Build history of the part. All positions in model axes, mm. A direction names the side the tool comes from. Round coordinates to 2 decimals unless told otherwise and drop trailing zeros. Loops run counter-clockwise (first coordinate to the right, second up) from the corner with the lowest first, then second, coordinate; pieces in that order, holes last. Notation, with made-up numbers: (53.25, 81) - (80.25, 81) arc R29 cw to (80.25, 118) - close; hole circle Ø6 at (67.5, 69). An arc over 180 degrees is marked (long way). Use a Markdown table: item, result.
from build123d import *

# Parameters (mm, degrees)
SKETCH2_W           = 60
SKETCH2_H           = 60
BOSS_EXTRUDE1_DEPTH = 15
CUT_EXTRUDE1_DEPTH  = 3
SKETCH1_R           = 2.25
BOSS_EXTRUDE2_DEPTH = 2
SKETCH4_R           = 1.25
BOSS_EXTRUDE3_DEPTH = 5
SKETCH5_R           = 2.5
BOSS_EXTRUDE4_DEPTH = 25


with BuildPart() as part:
    # Sketch2 → Boss-Extrude1 (new body)
    with BuildSketch(Plane(origin=(0, 0, 0), x_dir=(1, 0, 0), z_dir=(0, 1, 0))):
        Rectangle(SKETCH2_W, SKETCH2_H)
    extrude(amount=-BOSS_EXTRUDE1_DEPTH)

    # Sketch3 → Cut-Extrude1 (cut)
    with BuildSketch(Plane.ZY.offset(30)):
        with BuildLine():
            Line((-6.5, -7.5), (-13, -7.5))
            ThreePointArc((-13, -7.5), (-14.035987291, -9.767742066), (-16.428436053, -10.469249492))
            Line((-16.428436053, -10.469249492), (-4.5, -12.19041576))
            ThreePointArc((-4.5, -12.19041576), (-5.979130372, -10.049509757), (-6.5, -7.5))
        make_face()
        with BuildLine():
            ThreePointArc((-16.428436053, -10.469249492), (-14.035987291, -9.767742066), (-13, -7.5))
            Line((-13, -7.5), (-19, -7.5))
            ThreePointArc((-19, -7.5), (-18.267742066, -9.464012709), (-16.428436053, -10.469249492))
        make_face()
        with BuildLine():
            Line((-19, -7.5), (-13, -7.5))
            ThreePointArc((-13, -7.5), (-14.035987291, -5.232257934), (-16.428436053, -4.530750508))
            ThreePointArc((-16.428436053, -4.530750508), (-18.267742066, -5.535987291), (-19, -7.5))
        make_face()
        with BuildLine():
            ThreePointArc((-16.428436053, -4.530750508), (-14.035987291, -5.232257934), (-13, -7.5))
            Line((-13, -7.5), (-6.5, -7.5))
            ThreePointArc((-6.5, -7.5), (-5.979130372, -4.950490243), (-4.5, -2.80958424))
            Line((-4.5, -2.80958424), (-16.428436053, -4.530750508))
        make_face()
        with BuildLine():
            ThreePointArc((0, -12), (-3.18198051, -10.681980521), (-4.5, -7.500000016))
            Line((-4.5, -7.500000016), (-4.5, -12.19041576))
            ThreePointArc((-4.5, -12.19041576), (-2.425107994, -13.530659269), (0, -14))
            Line((0, -14), (0, -12))
        make_face()
        with BuildLine():
            Line((-4.5, -2.80958424), (-4.5, -7.500000016))
            ThreePointArc((-4.5, -7.500000016), (-3.181980521, -4.31801949), (0, -3))
            Line((0, -3), (0, -1))
            ThreePointArc((0, -1), (-2.425107994, -1.469340731), (-4.5, -2.80958424))
        make_face()
        with BuildLine():
            ThreePointArc((-4.5, -2.80958424), (-5.979130372, -4.950490243), (-6.5, -7.5))
            Line((-6.5, -7.5), (-4.5, -7.5))
            Line((-4.5, -7.500000016), (-4.5, -2.80958424))
        make_face()
        with BuildLine():
            Line((-4.5, -7.5), (-6.5, -7.5))
            ThreePointArc((-6.5, -7.5), (-5.979130372, -10.049509757), (-4.5, -12.19041576))
            Line((-4.5, -12.19041576), (-4.5, -7.500000016))
        make_face()
        with BuildLine():
            Line((0, -1), (0, -3))
            ThreePointArc((0, -3), (3.181980515, -4.318019485), (4.5, -7.5))
            Line((4.5, -7.5), (4.5, -2.80958424))
            ThreePointArc((4.5, -2.80958424), (2.425107994, -1.469340731), (0, -1))
        make_face()
        with BuildLine():
            ThreePointArc((4.5, -7.5), (3.181980515, -10.681980515), (0, -12))
            Line((0, -12), (0, -14))
            ThreePointArc((0, -14), (2.425107994, -13.530659269), (4.5, -12.19041576))
            Line((4.5, -12.19041576), (4.5, -7.5))
        make_face()
        with BuildLine():
            Line((0, -3), (0, -7.5))
            Line((0, -7.5), (4.5, -7.5))
            ThreePointArc((4.5, -7.5), (3.181980515, -4.318019485), (0, -3))
        make_face()
        with BuildLine():
            Line((4.5, -7.5), (0, -7.5))
            Line((0, -7.5), (0, -12))
            ThreePointArc((0, -12), (3.181980515, -10.681980515), (4.5, -7.5))
        make_face()
        with BuildLine():
            ThreePointArc((0, -3), (-3.181980521, -4.31801949), (-4.5, -7.500000016))
            Line((-4.5, -7.5), (0, -7.5))
            Line((0, -7.5), (0, -3))
        make_face()
        with BuildLine():
            Line((0, -7.5), (-4.5, -7.5))
            ThreePointArc((-4.5, -7.500000016), (-3.18198051, -10.681980521), (0, -12))
            Line((0, -12), (0, -7.5))
        make_face()
        with BuildLine():
            Line((4.5, -2.80958424), (4.5, -7.5))
            Line((4.5, -7.5), (6.5, -7.5))
            ThreePointArc((6.5, -7.5), (5.979130372, -4.950490243), (4.5, -2.80958424))
        make_face()
        with BuildLine():
            Line((6.5, -7.5), (4.5, -7.5))
            Line((4.5, -7.5), (4.5, -12.19041576))
            ThreePointArc((4.5, -12.19041576), (5.979130372, -10.049509757), (6.5, -7.5))
        make_face()
        with BuildLine():
            ThreePointArc((6.5, -7.5), (5.979130372, -10.049509757), (4.5, -12.19041576))
            Line((4.5, -12.19041576), (16.428436053, -10.469249492))
            ThreePointArc((16.428436053, -10.469249492), (14.035987291, -9.767742066), (13, -7.5))
            Line((13, -7.5), (6.5, -7.5))
        make_face()
        with BuildLine():
            Line((16.428436053, -4.530750508), (4.5, -2.80958424))
            ThreePointArc((4.5, -2.80958424), (5.979130372, -4.950490243), (6.5, -7.5))
            Line((6.5, -7.5), (13, -7.5))
            ThreePointArc((13, -7.5), (14.035987291, -5.232257934), (16.428436053, -4.530750508))
        make_face()
        with BuildLine():
            ThreePointArc((19, -7.5), (18.267742066, -5.535987291), (16.428436053, -4.530750508))
            ThreePointArc((16.428436053, -4.530750508), (14.035987291, -5.232257934), (13, -7.5))
            Line((13, -7.5), (19, -7.5))
        make_face()
        with BuildLine():
            ThreePointArc((13, -7.5), (14.035987291, -9.767742066), (16.428436053, -10.469249492))
            ThreePointArc((16.428436053, -10.469249492), (18.267742066, -9.464012709), (19, -7.5))
            Line((19, -7.5), (13, -7.5))
        make_face()
    extrude(amount=-CUT_EXTRUDE1_DEPTH, mode=Mode.SUBTRACT)

    # Sketch1 → Boss-Extrude2 (add)
    with BuildSketch(Plane(origin=(0, 0, 0), x_dir=(1, 0, 0), z_dir=(0, 1, 0))):
        with Locations(Location((-23.4, -8.623991148, 0), (0, 0, 90))):
            Circle(SKETCH1_R)
        with Locations(Location((0, 23.296008852, 0), (0, 0, 90))):
            Circle(SKETCH1_R)
        with Locations(Location((23.4, -8.623991148, 0), (0, 0, 90))):
            Circle(SKETCH1_R)
    extrude(amount=BOSS_EXTRUDE2_DEPTH)

    # Sketch4 → Boss-Extrude3 (add)
    with BuildSketch(Plane(origin=(0, 2, 0), x_dir=(1, 0, 0), z_dir=(0, 1, 0))):
        with Locations(Location((-23.4, -8.623991148, 0), (0, 0, 270))):
            Circle(SKETCH4_R)
        with Locations(Location((23.4, -8.623991148, 0), (0, 0, 270))):
            Circle(SKETCH4_R)
        with Locations(Location((0, 23.296008852, 0), (0, 0, 270))):
            Circle(SKETCH4_R)
    extrude(amount=BOSS_EXTRUDE3_DEPTH)

    # Sketch5 → Boss-Extrude4 (add)
    with BuildSketch(Plane(origin=(30, 0, 0), x_dir=(0, 0, -1), z_dir=(1, 0, 0))):
        with Locations((0, -7.5)):
            Circle(SKETCH5_R)
    extrude(amount=BOSS_EXTRUDE4_DEPTH)


solid = part.part
Q1. Probe line 1 (Y direction, x = 10, z = 27.5); line 2 (X direction, y = -1.5, z = -20); line 3 (X direction, y = -9.25, z = -13). List the from-to ranges inside material, lowest first.
Results found:
| item | result |
|---|---|
| line 1 | y = -15 to 0 |
| line 2 | x = -30 to 30 |
| line 3 | x = -27 to 30 |
Q2. Cut at D-D, the plane x = 47. List the corners of the cut face in (y, z).
Results found:
| item | result |
|---|---|
| outline | circle Ø5 at (-7.5, 0) |
Q3. Pull direction Y, two halves, no side cores. Call faces 1 (the face through (-22, 2, 8)), 2 (the face through (42.32, -9.94, 0.54)), 3 (the face through (0, -7, -30)), 4 (the face through (-28.52, -3.66, -10.38)): pulls with the +Y half, pulls with the -Y half, needs draft (parallel to the pull), parting line crosses it, or undercut.
Results found:
| item | result |
|---|---|
| face 1 | pulls with the +Y half |
| face 2 | parting line crosses it |
| face 3 | needs draft |
| face 4 | undercut |
Q4. Cut at A-A, the plane x = -23.4. List the corners of the cut face in (y, z).
Results found:
| item | result |
|---|---|
| outline | (-15, -30) - (0, -30) - (0, 6.37) - (2, 6.37) - (2, 7.37) - (7, 7.37) - (7, 9.87) - (2, 9.87) - (2, 10.87) - (0, 10.87) - (0, 30) - (-15, 30) - close |
Q5. Drop flat-ended pins along their axis: pin 1 (1.5 mm diameter, centred on x = 26, y = 1.5, fed in from +Z); pin 2 (10 mm diameter, centred on y = 0.5, z = 8.5, fed in from +X); pin 3 (4 mm diameter, centred on y = -5.5, z = 4.5, fed in from -X); pin 4 (4 mm diameter, centred on y = 0.5, z = 20, fed in from -X). Give the stop position or say it passes through.
Results found:
| item | result |
|---|---|
| pin 1 | stops at z = 9.9 |
| pin 2 | stops at x = 30 |
| pin 3 | stops at x = -27 |
| pin 4 | stops at x = -30 |
Q6. Which spindle directions (+Z, -Z, +X, -X, +Y, -Y) get a long thin tool onto all of the face, cutting with end or side? Do faces 5 (the face through (-28.521, -3.682, 10.548)), 6 (the face through (55, -7, 0)), 7 (the face through (-0.48, 4.46, -22.14)). Say none if no direction does.
Results found:
| item | result |
|---|---|
| face 5 | -X |
| face 6 | +Z, -Z, +X, +Y, -Y |
| face 7 | +Y |
Q7. Cut at B-B, the plane y = -6.25. List the corners of the cut face in (x, z).
Results found:
| item | result |
|---|---|
| outline | (-30, -30) - (30, -30) - (30, -2.17) - (55, -2.17) - (55, 2.17) - (30, 2.17) - (30, 30) - (-30, 30) - (-30, 18.73) - (-27, 18.73) - (-27, -18.73) - (-30, -18.73) - close |
Q8. Cut at C-C, the plane z = 12. List the corners of the cut face in (x, y), plus the area to 3 significant figures.
Results found:
| item | result |
|---|---|
| outline | (-30, -15) - (30, -15) - (30, 0) - (-30, 0) - (-30, -3.89) - (-27, -3.89) - (-27, -11.11) - (-30, -11.11) - close |
| area | 878 mm2 |
